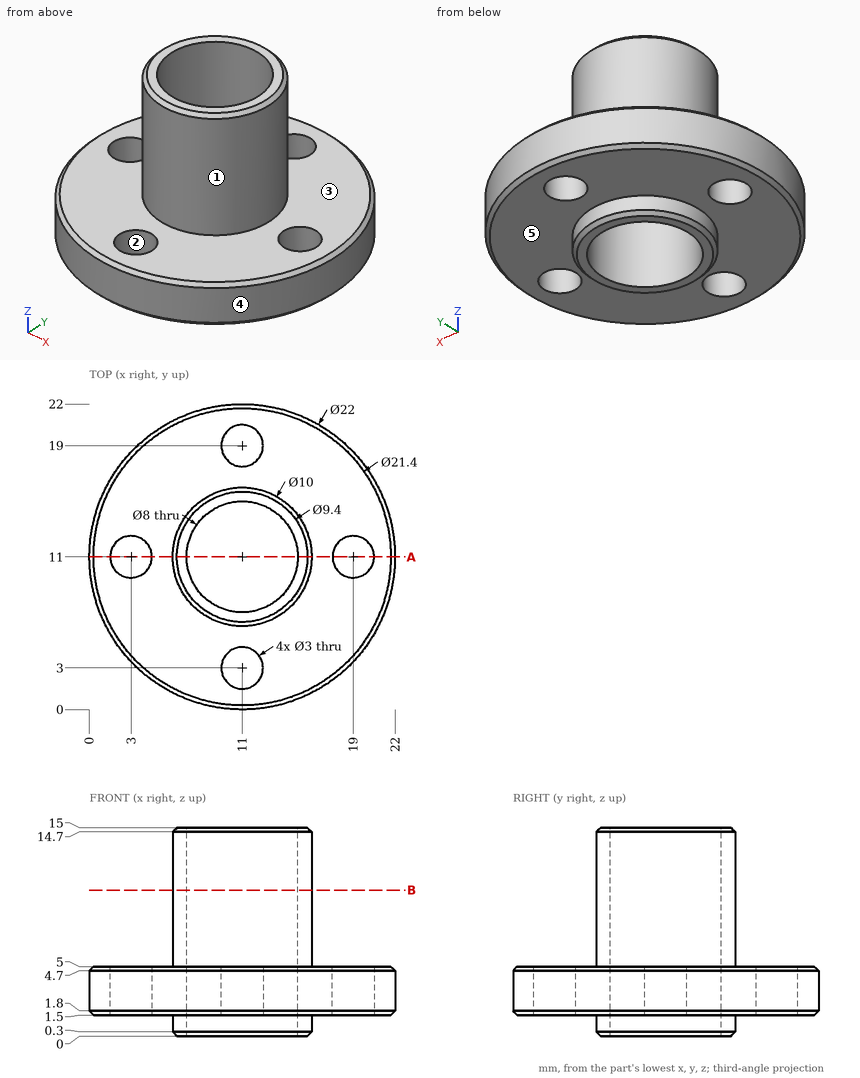
Answer from the drawing. Dimensions are ordinates in mm from the lowest x, y and z of the part. A direction names the side the tool comes from. Coordinates: 2 decimals unless noted, no trailing zeros. Order: outer loops, then holes, each group sorted by start corner. A loop starts at its lowest first (then second) coordinate and runs counter-clockwise, first axis right, second up. Notation, with made-up numbers: M -17.75,-25.75 L 4.25,-25.75 A24 ccw 4.25,-13.75 Z; hole C -39.75,4.25 d11. An arc over 180 degrees is marked long. Put each result on its own line as item: value. Start each with the question number.
Item 1: The mould has two halves that part along X. Classify the marked faces 1, 2 and 3: +X half, -X half, draft (parallel to the pull), parting line (faces both ways), or undercut.
Item 2: Given pin 1 Ø1 at (y, z) = (15, 12.5) entering from +X; pin 2 Ø3 at (x, y) = (13.5, 4) entering from -Z; pin 3 Ø2.5 at (x, y) = (11, 19) entering from +Z; pin 4 Ø12 at (x, y) = (19, 6.5) entering from -Z, each flat-ended and moving along its own axis, determine where each tip first touches the part or whether it passes through.
Item 3: Section A-A, the plane y = 11 is taken. Count the separate pieces of the cut face and the enclosed holes in it, plus the area to 3 significant figures.
Item 4: Consider probe 1 along Y at (x, z) = (11, 3.5); probe 2 along Y at (x, z) = (11, 7.25); probe 3 along Z at (x, y) = (9.25, 20.5). Determine where each line is inside the solid, lowest interval first. Write a range as [from, to].
Item 5: Section B-B, the plane z = 10.5 is taken. Determine the outline of the cut face in (x, y), plus the area to 3 significant figures.
Item 6: For the marked faces 4 and 5, determine the directions among +Z, -Z, +X, -X, +Y, -Y from which every point of the face is accessible in a straight line to the end or side of a thin tool.
Computed:
1. face 1: parting line
1. face 2: undercut
1. face 3: draft
2. pin 1: stops at x = 14.57
2. pin 2: stops at z = 1.5
2. pin 3: passes through
2. pin 4: stops at z = 0
3. separate pieces: 4
3. enclosed holes: 0
3. area: 50.6 mm2
4. probe 1: y = [0, 1.5], [4.5, 7], [15, 17.5], [20.5, 22]
4. probe 2: y = [6, 7], [15, 16]
4. probe 3: z = [1.5, 5]
5. outline: C 11,11 d10; hole C 11,11 d8
5. area: 28.3 mm2
6. face 4: +Z, -Z
6. face 5: -Z
